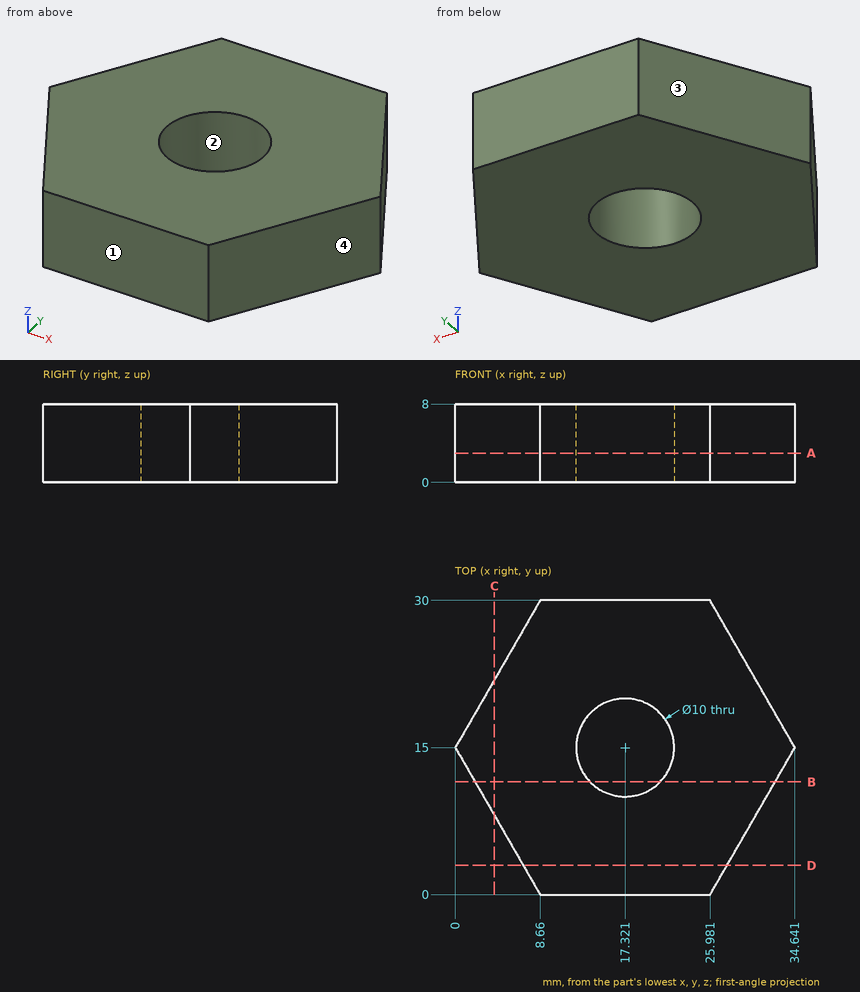
Geometry check sheet. Reference: drawing and pictorial views, mm from the part's lowest x, y, z. Coordinates: 2 decimals unless noted, no trailing zeros. Loops run counter-clockwise (first coordinate to the right, second up) from the corner with the lowest first, then second, coordinate; pieces in that order, holes last. Notation, with made-up numbers: (-36, -1.5) - (-5, -1.5) arc R19 cw to (-5, 11.5) - close; hole circle Ø6 at (-26, 33.25). An arc over 180 degrees is marked (long way). Return JSON: item names as keys, results as strings.
1. Go/stop test with flat-tipped pins: pin 1 (8 mm diameter, centred on x = 17.32, y = 15, fed in from +Z); pin 2 (2 mm diameter, centred on y = 23.5, z = 6, fed in from -X). Record where each tip stops, or that it passes through.
Established:
{"pin 1": "passes through", "pin 2": "stops at x = 4.33"}
2. Mould release check, pull along X, two halves, no side actions. Record for the marked faces 1, 2, 3 and 4: +X half, -X half, draft (parallel to the pull), parting line (faces both ways), or undercut.
Established:
{"face 1": "draft", "face 2": "undercut", "face 3": "-X half", "face 4": "+X half"}
3. Section check B-B, the plane y = 11.5. Record the boundary of the cut face in (x, z).
Established:
{"outline": "(2.02, 0) - (13.75, 0) - (13.75, 8) - (2.02, 8) - close; (20.89, 0) - (32.62, 0) - (32.62, 8) - (20.89, 8) - close"}
4. Section check C-C, the plane x = 4. Record the boundary of the cut face in (y, z).
Established:
{"outline": "(8.07, 0) - (21.93, 0) - (21.93, 8) - (8.07, 8) - close"}
5. Section check A-A, the plane z = 3. Record the boundary of the cut face in (x, y), then the cut area to 3 significant figures.
Established:
{"outline": "(0, 15) - (8.66, 0) - (25.98, 0) - (34.64, 15) - (25.98, 30) - (8.66, 30) - close; hole circle Ø10 at (17.32, 15)", "area": "701 mm2"}
6. Section check D-D, the plane y = 3. Record the boundary of the cut face in (x, z).
Established:
{"outline": "(6.93, 0) - (27.71, 0) - (27.71, 8) - (6.93, 8) - close"}
7. Thickness scan on L1, parallel to Y at x = 19.5, z = 5; L2, parallel to X at y = 18, z = 1; L3, parallel to X at y = 18.25, z = 7 (1 decimal). Record the ranges inside material, lowest first.
Established:
{"L1": "y = 0 to 10.5, 19.5 to 30", "L2": "x = 1.73 to 13.32, 21.32 to 32.91", "L3": "x = 1.9 to 13.5, 21.1 to 32.8"}
